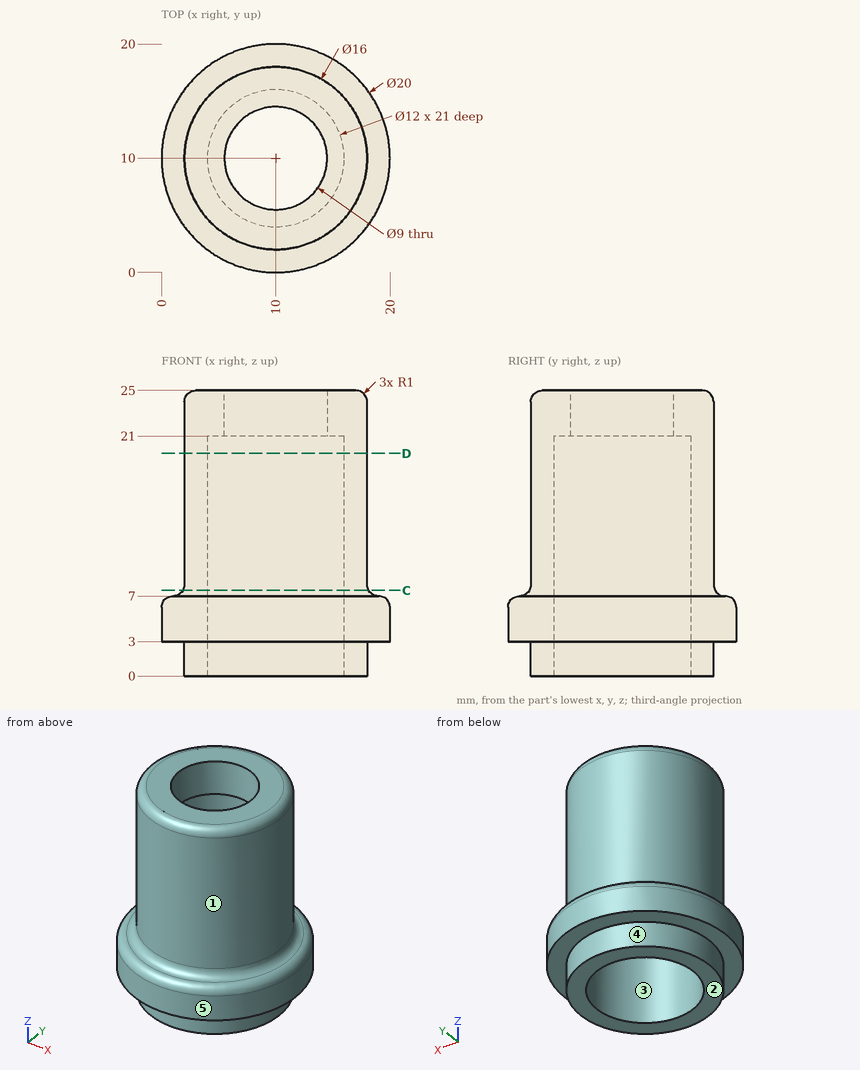
Job drawing, mm, ordinate dimensions from the low corner. One solid piece. A direction names the side the tool comes from. Round coordinates to 2 decimals unless told otherwise and drop trailing zeros. Loops run counter-clockwise (first coordinate to the right, second up) from the corner with the lowest first, then second, coordinate; pieces in that order, holes last. Notation, with made-up numbers: M 40.5,64 L 87.5,64 A22 cw 87.5,100 Z; hole C 52.5,48 d9. An arc over 180 degrees is marked long. One line per question, with ' | ' between items. Start each with the question number.
Item 1: Two-plate mould, pull along X, no slides. Class the marked faces 1, 2 and 3: pulls with the +X half, pulls with the -X half, needs draft (parallel to the pull), parting line crosses it, or undercut.
Item 2: Cut at C-C, the plane z = 7.5. Write the cut outline in (x, y), plus the area to 3 significant figures.
Item 3: Pin check, flat tips, straight feed: pin 1 Ø5 at (x, z) = (4.5, 14.5) entering from -Y; pin 2 Ø12 at (y, z) = (3.5, 15.5) entering from -X; pin 3 Ø1.5 at (x, y) = (12.5, 7) entering from -Z; pin 4 Ø7 at (x, y) = (10, 10) entering from +Z. Stop position of each tip, or through.
Item 4: Wall check: line 1 (Y direction, x = 10, z = 14); line 2 (Y direction, x = 10, z = 22.4); line 3 (Z direction, x = 6, y = 12.75). Give the ranges that are in metal, low to high.
Item 5: Which spindle directions (+Z, -Z, +X, -X, +Y, -Y) get a long thin tool onto all of the face, cutting with end or side? Do the marked faces 4 and 5. Say none if no direction does.
Item 6: Cut at D-D, the plane z = 19.5. Write the cut outline in (x, y).
Responses:
1) face 1: parting line crosses it | face 2: needs draft | face 3: undercut
2) outline: C 10,10 d16.27; hole C 10,10 d12 | area: 94.8 mm²
3) pin 1: stops at y = 2.58 | pin 2: stops at x = 2.02 | pin 3: stops at z = 21 | pin 4: passes through
4) line 1: y = 2 to 4, 16 to 18 | line 2: y = 2 to 5.5, 14.5 to 18 | line 3: z = 21 to 25
5) face 4: -Z | face 5: +Z, -Z
6) outline: C 10,10 d16; hole C 10,10 d12
